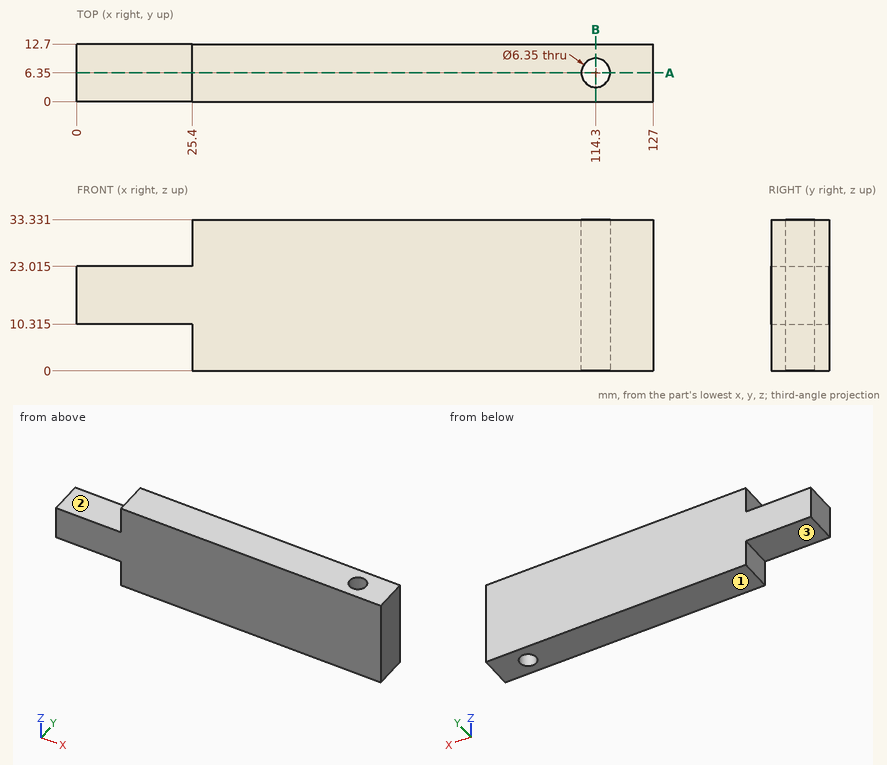
Print and shaded views of the part. All mm, measured from the part's lowest x, y and z. A direction names the side the tool comes from. Coordinates: 2 decimals unless noted, no trailing zeros. Order: outer loops, then holes, each group sorted by start corner. A loop starts at its lowest first (then second) coordinate and runs counter-clockwise, first axis right, second up. Notation, with made-up numbers: (54.5, 27.25) - (61.5, 27.25) arc R29 cw to (61.5, 49.25) - close; hole circle Ø11 at (22, 43). An arc over 180 degrees is marked (long way). Put each result on its own line as item: value.
1. Drop a flat-ended pin along its axis: P1, Ø4, axis at y = 4, z = 25.5, coming from the -X side. Give the stop position or say it passes through.
Answer sheet:
P1: stops at x = 25.4
2. Probe line 1 along Y through (x, z) = (114.3, 23) (1 decimal); line 2 along X through (y, z) = (5.75, 20); line 3 along X through (y, z) = (7.75, 25). List the from-to ranges inside material, lowest first. Write a range as [from, to].
Answer sheet:
line 1: y = [0, 3.2], [9.5, 12.7]
line 2: x = [0, 111.18], [117.42, 127]
line 3: x = [25.4, 111.45], [117.15, 127]
3. Tool access for the marked faces 1, 2 and 3: list every direction of +Z, -Z, +X, -X, +Y, -Y with a clear straight run to the whole face (end or side of a thin tool).
Answer sheet:
face 1: -Z, +X, -X, +Y, -Y
face 2: +Z, -X, +Y, -Y
face 3: -Z, -X, +Y, -Y
4. Saw through at A-A (y = 6.35). Write the cut outline in (x, z) (1 decimal).
Answer sheet:
outline: (0, 10.3) - (25.4, 10.3) - (25.4, 0) - (111.1, 0) - (111.1, 33.3) - (25.4, 33.3) - (25.4, 23) - (0, 23) - close; (117.5, 0) - (127, 0) - (127, 33.3) - (117.5, 33.3) - close
5. Saw through at B-B (x = 114.3). Write the cut outline in (y, z) (1 decimal), and give its area (3 significant figures).
Answer sheet:
outline: (0, 0) - (3.2, 0) - (3.2, 33.3) - (0, 33.3) - close; (9.5, 0) - (12.7, 0) - (12.7, 33.3) - (9.5, 33.3) - close
area: 212 mm^2
